Verification items for the finished model (mm, model axes). A direction names the side the tool comes from. Round coordinates to 2 decimals unless told otherwise and drop trailing zeros. Write each loop counter-clockwise with the first axis right and the second up, starting at its lowest first coordinate (ties: lowest second). Pieces come first, ordered by that corner, then holes. Notation, with made-up numbers: (50, 54) - (69, 54) arc R26 ccw to (69, 91) - close; hole circle Ø4 at (69, 56). An arc over 180 degrees is marked (long way). Answer as a JSON object with one key per item and string values. Group by question number.
1) Section check C-C (y = 22). Enter the section's corners in (x, z).
2) Mould release check, pull along Z, two halves, no side actions. Record for faces 6 (the cylindrical face through (13.1, -39, -11.9)), 7 (the flat face through (11.3, -40, 11.3)), 8 (the flat face through (21, 99, 2.214)), 9 (the cylindrical face through (13.1, -39, 11.9)): +Z half, -Z half, draft (parallel to the pull), parting line (faces both ways), or undercut.
3) Set-up check for faces 1 (the cylindrical face through (-13.1, -39, 11.9)), 2 (the flat face through (13, -38, -11)), 3 (the flat face through (-13, -38, -11)), 4 (the flat face through (-12.2, -38, 11.4)), 5 (the cylindrical face through (-13.1, -39, -11.9)): record each of +Z, -Z, +X, -X, +Y, -Y from which the full face is reachable in a straight line by a thin tool's end or side.
4) Go/stop test with flat-tipped pins: pin 1 Ø5 at (x, y) = (16, 5.5) entering from -Z; pin 2 Ø1.5 at (x, y) = (5.5, 133) entering from +Z; pin 3 Ø6.5 at (x, y) = (17, 109) entering from -Z. Record where each tip stops, or that it passes through.
5) Thickness scan on line 1 (Z direction, x = 0, y = 64.5); line 2 (Y direction, x = 6, z = -14.5); line 3 (Y direction, x = 10, z = -14). Record the ranges inside material, lowest first.
6) Section check A-A (x = 11). Enter the section's corners in (y, z), then the cut area to 3 significant figures.
7) Section check B-B (z = 12). Enter the section's corners in (x, y).
```python
from build123d import *

# Parameters (mm, degrees)
SKETCH1_R           = 21.59
BOSS_EXTRUDE1_DEPTH = 200
SHELL1_T            = 2
CUT_EXTRUDE1_START  = 20
CUT_EXTRUDE1_DEPTH  = 5
SKETCH4_R           = 16.5
BOSS_EXTRUDE2_DEPTH = 40
SKETCH7_R           = 15.5
CUT_EXTRUDE4_DEPTH  = 62
SKETCH8_W           = 2.785852998
SKETCH8_H           = 5.87658936
SKETCH8_W_2         = 8.878050256
SKETCH8_H_2         = 3.207420782
SKETCH8_W_3         = 2.758641046
SKETCH8_H_3         = 8.505589864
CUT_EXTRUDE5_DEPTH  = 203.317216766
BOSS_EXTRUDE4_DEPTH = 2
SKETCH10_R          = 21.59
CUT_EXTRUDE7_DEPTH  = 2.5


with BuildPart() as part:
    # Sketch1 → Boss-Extrude1 (new body)
    with BuildSketch(Plane(origin=(0, 0, 0), x_dir=(1, 0, 0), z_dir=(0, 1, 0))):
        with Locations(Location((0, 0, 0), (0, 0, 270))):
            Circle(SKETCH1_R)
    extrude(amount=BOSS_EXTRUDE1_DEPTH)

    # Shell1 (no face opened: a closed hollow body)
    add(offset(amount=-SHELL1_T, mode=Mode.PRIVATE), mode=Mode.SUBTRACT)

    # Sketch2 → Cut-Extrude1 (cut, symmetric)
    with BuildSketch(Plane(origin=(0, 0, 0), x_dir=(0, 0, -1), z_dir=(1, 0, 0)).offset(CUT_EXTRUDE1_START)):
        Polygon((2.213988381, 104.269834735), (2.213988381, 0), (-2.213988381, 0), (-2.213988381, 104.269834735), (-2.213988381, 199.79439609), (2.213988381, 199.79439609), align=None)
    extrude(amount=CUT_EXTRUDE1_DEPTH, both=True, mode=Mode.SUBTRACT)

    # Sketch4 → Boss-Extrude2 (add)
    with BuildSketch(Plane.XZ):
        with Locations(Location((0, 0, 0), (0, 0, 7.711270357))):
            Circle(SKETCH4_R)
    extrude(amount=BOSS_EXTRUDE2_DEPTH)

    # Sketch7 → Cut-Extrude4 (cut)
    with BuildSketch(Plane(origin=(0, -40, 0), x_dir=(-1, 0, 0), z_dir=(0, -1, 0))):
        with Locations(Location((0, 0, 0), (0, 0, 90))):
            Circle(SKETCH7_R)
    extrude(amount=-CUT_EXTRUDE4_DEPTH, mode=Mode.SUBTRACT)

    # Sketch8 → Cut-Extrude5 (cut, through all)
    with BuildSketch(Plane(origin=(0, 0, 0), x_dir=(1, 0, 0), z_dir=(0, 1, 0))):
        with Locations((0, 20.108138302)):
            Rectangle(SKETCH8_W, SKETCH8_H)
        with Locations((18.709836445, -0.001004202)):
            Rectangle(SKETCH8_W_2, SKETCH8_H_2)
        with Locations((0.013605976, -18.452209414)):
            Rectangle(SKETCH8_W_3, SKETCH8_H_3)
        with Locations((-18.709836445, -0.001004202)):
            Rectangle(SKETCH8_W_2, SKETCH8_H_2)
    extrude(amount=-CUT_EXTRUDE5_DEPTH, mode=Mode.SUBTRACT)

    # Sketch9 → Boss-Extrude4 (add)
    with BuildSketch(Plane.XZ.offset(40)):
        with BuildLine():
            ThreePointArc((16.726333299, 4.561841417), (13.056013579, 11.944688127), (5.932226465, 16.095510881))
            ThreePointArc((5.932226465, 16.095510881), (5.137631387, 15.609709062), (5.623433206, 14.815113985))
            ThreePointArc((5.623433206, 14.815113985), (12.094357446, 11.044695365), (15.428308962, 4.338453169))
            ThreePointArc((15.428308962, 4.338453169), (16.189015254, 3.801135125), (16.726333299, 4.561841417))
        make_face()
        with BuildLine():
            ThreePointArc((16.726333299, -4.561841417), (13.056013579, -11.944688127), (5.932226465, -16.095510881))
            ThreePointArc((5.932226465, -16.095510881), (5.137631387, -15.609709062), (5.623433206, -14.815113985))
            ThreePointArc((5.623433206, -14.815113985), (12.094357446, -11.044695365), (15.428308962, -4.338453169))
            ThreePointArc((15.428308962, -4.338453169), (16.189015254, -3.801135125), (16.726333299, -4.561841417))
        make_face()
        with BuildLine():
            ThreePointArc((-16.726333299, -4.561841417), (-13.056013579, -11.944688127), (-5.932226465, -16.095510881))
            ThreePointArc((-5.932226465, -16.095510881), (-5.137631387, -15.609709062), (-5.623433206, -14.815113985))
            ThreePointArc((-5.623433206, -14.815113985), (-12.094357446, -11.044695365), (-15.428308962, -4.338453169))
            ThreePointArc((-15.428308962, -4.338453169), (-16.189015254, -3.801135125), (-16.726333299, -4.561841417))
        make_face()
        with BuildLine():
            ThreePointArc((-16.726333299, 4.561841417), (-13.056013579, 11.944688127), (-5.932226465, 16.095510881))
            ThreePointArc((-5.932226465, 16.095510881), (-5.137631387, 15.609709062), (-5.623433206, 14.815113985))
            ThreePointArc((-5.623433206, 14.815113985), (-12.094357446, 11.044695365), (-15.428308962, 4.338453169))
            ThreePointArc((-15.428308962, 4.338453169), (-16.189015254, 3.801135125), (-16.726333299, 4.561841417))
        make_face()
    extrude(amount=-BOSS_EXTRUDE4_DEPTH)

    # Sketch10 → Cut-Extrude7 (cut, symmetric)
    with BuildSketch(Plane(origin=(0, 200, 0), x_dir=(1, 0, 0), z_dir=(0, 1, 0))):
        Circle(SKETCH10_R)
    extrude(amount=CUT_EXTRUDE7_DEPTH, both=True, mode=Mode.SUBTRACT)


solid = part.part
```
Returned:
{
 "1": {"outline": "(19.46, -2.21) arc R19.59 cw (long way) to (19.46, 2.21) - (21.48, 2.21) arc R21.59 ccw (long way) to (21.48, -2.21) - close"},
 "2": {"face 6": "-Z half", "face 7": "draft", "face 8": "undercut", "face 9": "+Z half"},
 "3": {"face 1": "+Z, -X, -Y", "face 2": "-Z, +X", "face 3": "-Z, -X", "face 4": "+Z, -X", "face 5": "-Z, -X, -Y"},
 "4": {"pin 1": "z = -16.85", "pin 2": "z = 21.06", "pin 3": "z = -16.65"},
 "5": {"line 1": "-21.59 to -19.59, 19.59 to 21.59", "line 2": "-40 to 2", "line 3": "-40 to -38, 0 to 2"},
 "6": {"outline": "(-40, -13.76) - (-38, -13.76) - (-38, -12.3) - (0, -12.3) - (0, -18.58) - (197.5, -18.58) - (197.5, -16.21) - (2, -16.21) - (2, -10.92) - (-40, -10.92) - close; (-40, 10.92) - (2, 10.92) - (2, 16.21) - (197.5, 16.21) - (197.5, 18.58) - (0, 18.58) - (0, 12.3) - (-38, 12.3) - (-38, 13.76) - (-40, 13.76) - close", "area": "1,070 mm2"},
 "7": {"outline": "(-17.95, 0) - (-11.32, 0) - (-11.32, -38) - (-13, -38) - (-13, -40) - (-9.81, -40) - (-9.81, 2) - (-15.48, 2) - (-15.48, 197.5) - (-17.95, 197.5) - close; (9.81, -40) - (13, -40) - (13, -38) - (11.32, -38) - (11.32, 0) - (17.95, 0) - (17.95, 197.5) - (15.48, 197.5) - (15.48, 2) - (9.81, 2) - close"}
}
